For this review, take the finished solid that the model builds, in its own axes (mm). A direction names the side the tool comes from. Coordinates: 2 decimals unless noted, no trailing zeros. Loops run counter-clockwise (first coordinate to the right, second up) from the corner with the lowest first, then second, coordinate; pieces in that order, holes last. Notation, with made-up numbers: (26, 85) -> (64, 85) arc R19 cw to (64, 118) -> close; hole circle Ø11 at (63, -35.5). An arc over 180 degrees is marked (long way). One line per item, written item: value.
from build123d import *

# Parameters (mm, degrees)
BOSS_EXTRUDE2_DEPTH = 1.5875
CUT_EXTRUDE4_DEPTH  = 216.037664516
FILLET4_R           = 2.54
SKETCH8_W           = 25.4
SKETCH8_H           = 1.5875
CUT_EXTRUDE5_DEPTH  = 216.037664516


with BuildPart() as part:
    # Sketch6 → Boss-Extrude2 (new body)
    with BuildSketch(Plane.XY):
        Polygon((63.5, 12.997971671), (63.5, -205.442028329), (-30.988, -205.442028329), (0, 14.585471671), (38.1, 14.585471671), (38.1, 12.997971671), align=None)
    extrude(amount=BOSS_EXTRUDE2_DEPTH)

    # Sketch7 → Cut-Extrude4 (cut, through all)
    with BuildSketch(Plane.XY.offset(1.5875)):
        Polygon((-14.078119511, -176.440074821), (43.990131885, -95.296788202), (8.777825003, -14.153501583), align=None)
        Polygon((-7.003851095, -192.742028329), (52.698191605, -109.315717977), (52.698191605, -192.742028329), align=None)
        Polygon((52.698191605, -77.080404102), (19.119676028, 0.297971671), (52.698191605, 0.297971671), align=None)
    extrude(amount=-CUT_EXTRUDE4_DEPTH, mode=Mode.SUBTRACT)

    # Fillet4
    fillet4_edges = [part.edges().sort_by_distance(p)[0] for p in [
        (52.698191605, -109.315717977, 0.79375),
        (52.698191605, -192.742028329, 0.79375),
        (-7.003851095, -192.742028329, 0.79375),
        (-14.078119511, -176.440074821, 0.79375),
        (8.777825003, -14.153501583, 0.79375),
        (43.990131885, -95.296788202, 0.79375),
        (52.698191605, 0.297971671, 0.79375),
        (52.698191605, -77.080404102, 0.79375),
        (19.119676028, 0.297971671, 0.79375),
    ]]
    fillet(fillet4_edges, radius=FILLET4_R)

    # Sketch8 → Cut-Extrude5 (cut, through all)
    with BuildSketch(Plane.XY.offset(1.5875)):
        with Locations((50.8, -204.648278329)):
            Rectangle(SKETCH8_W, SKETCH8_H)
    extrude(amount=-CUT_EXTRUDE5_DEPTH, mode=Mode.SUBTRACT)


solid = part.part
1. Insertion check: pin 1 Ø0.5 at (x, z) = (50, 1) entering from +Y; pin 2 Ø0.8 at (y, z) = (-205, 1) entering from +X; pin 3 Ø0.5 at (y, z) = (-137.5, 0.5) entering from -X. Each pin has a flat end and moves straight along its axis. Give the tip position at first contact, or say it passes through.
Return value:
pin 1: stops at y = 13
pin 2: stops at x = 38.1
pin 3: stops at x = -21.45
2. Take a section at B-B, the plane y = -70. Give the boundary of the cut face in (x, z), and give its area (3 significant figures).
Return value:
outline: (-11.91, 0) -> (0.91, 0) -> (0.91, 1.59) -> (-11.91, 1.59) -> close; (33.01, 0) -> (63.5, 0) -> (63.5, 1.59) -> (33.01, 1.59) -> close
area: 68.8 mm2
3. Take a section at C-C, the plane x = 2. Give the boundary of the cut face in (y, z).
Return value:
outline: (-205.44, 0) -> (-192.74, 0) -> (-192.74, 1.59) -> (-205.44, 1.59) -> close; (-180.16, 0) -> (-153.97, 0) -> (-153.97, 1.59) -> (-180.16, 1.59) -> close; (-62.28, 0) -> (14.59, 0) -> (14.59, 1.59) -> (-62.28, 1.59) -> close
4. Take a section at A-A, the plane z = 0.5. Give the boundary of the cut face in (x, y), and give its area (3 significant figures).
Return value:
outline: (-30.99, -205.44) -> (38.1, -205.44) -> (38.1, -203.85) -> (63.5, -203.85) -> (63.5, 13) -> (38.1, 13) -> (38.1, 14.59) -> (0, 14.59) -> close; hole (-12.63, -166.19) arc R2.54 ccw to (-8.05, -168.02) -> (43.15, -96.47) arc R2.54 ccw to (43.42, -93.98) -> (12.37, -22.42) arc R2.54 ccw to (7.52, -23.08) -> close; hole (-4.13, -188.72) arc R2.54 ccw to (-2.06, -192.74) -> (50.16, -192.74) arc R2.54 ccw to (52.7, -190.2) -> (52.7, -117.23) arc R2.54 ccw to (48.09, -115.75) -> close; hole (20.66, -3.25) -> (47.83, -65.86) arc R2.54 ccw to (52.7, -64.85) -> (52.7, -2.24) arc R2.54 ccw to (50.16, 0.3) -> (22.99, 0.3) arc R2.54 ccw to start
area: 9,800 mm2
5. To check wall thickness, follow probe 1 along Y at (x, z) = (37.5, 1.4); probe 2 along Y at (x, z) = (18, 1.15); probe 3 along Y at (x, z) = (39, 0.3). State the ranges of each line that lie inside material, in increasing order. Write a range as from..to.
Return value:
probe 1: y = -205.44..-192.74, -130.55..-104.37, -80.34..-42.06, 0.3..14.59
probe 2: y = -205.44..-192.74, -157.8..-131.61, -35.41..14.59
probe 3: y = -203.85..-192.74, -128.46..-102.27, -83.8..-45.51, 0.3..13
6. Take a section at D-D, the plane y = -128. Give the boundary of the cut face in (x, z).
Return value:
outline: (-20.08, 0) -> (-7.26, 0) -> (-7.26, 1.59) -> (-20.08, 1.59) -> close; (20.59, 0) -> (39.33, 0) -> (39.33, 1.59) -> (20.59, 1.59) -> close; (52.7, 0) -> (63.5, 0) -> (63.5, 1.59) -> (52.7, 1.59) -> close
7. The part is to be moulded in two halves that separate along Y. For faces 1 (the flat face through (28.11, -58.7, 0.8)), 2 (the flat face through (-15.71, -96.97, 0.78)), 3 (the flat face through (38, -69, 0)), say which applies: pulls with the +Y half, pulls with the -Y half, needs draft (parallel to the pull), parting line crosses it, or undercut.
Return value:
face 1: undercut
face 2: pulls with the +Y half
face 3: needs draft
8. For faces 4 (the flat face through (-2.416, -93.632, 0.805)), 5 (the flat face through (38, -69, 1.588)), list the 3-axis set-ups (+Z, -Z, +X, -X, +Y, -Y) from which the entire face can be reached by the end or side of a thin tool; tool diameter is ignored.
Return value:
face 4: +Z, -Z
face 5: +Z, +X, -X, +Y, -Y
